The model under review builds one solid part; all positions refer to its coordinate system, in mm. Face numbers are marked on the shaded views. A direction names the side the tool comes from. Round coordinates to 2 decimals unless told otherwise and drop trailing zeros. Order: outer loops, then holes, each group sorted by start corner. A loop starts at its lowest first (then second) coordinate and runs counter-clockwise, first axis right, second up. Notation, with made-up numbers: M -34,43.25 L 0,43.25 A30 ccw 0,68.25 Z; hole C 45,-17.5 d2. An arc over 180 degrees is marked long. Use a Markdown table: item, result. Add a question column.
1. Insertion check: P1, Ø7, axis at x = -29, y = 60.5, coming from the +Z side; P2, Ø1, axis at x = -13, y = 155, coming from the -Z side; P3, Ø6.5, axis at x = 2.5, z = -15.5, coming from the +Y side; P4, Ø4, axis at y = 92, z = -23.5, coming from the -X side (1 decimal). Each pin has a flat end and moves straight along its axis. Give the tip position at first contact, or say it passes through.
2. Consider section A-A on y = 153. State the section outline as (x, z) points, then the cut area to 3 significant figures.
3. Consider section B-B on z = 17. State the section outline as (x, y) points, then the cut area to 3 significant figures.
4. For the marked faces 1, 2 and 3, list the 3-axis set-ups (+Z, -Z, +X, -X, +Y, -Y) from which the entire face can be reached by the end or side of a thin tool; tool diameter is ignored.
5. Consider section D-D on z = 0. State the section outline as (x, y) points.
6. Consider section C-C on x = 21.5. State the section outline as (y, z) points.
7. To check wall thickness, follow probe 1 along X at (y, z) = (41.5, 0); probe 2 along Y at (x, z) = (24.5, -16); probe 3 along Z at (x, y) = (0, 85). State the ranges of each line that lie inside material, in increasing order.
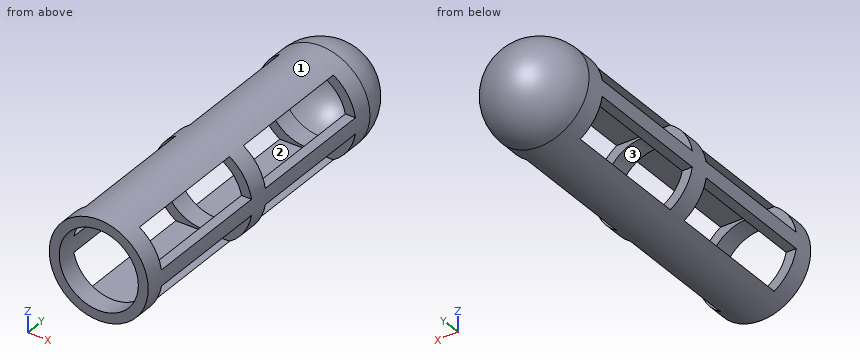
from build123d import *

# Parameters (mm, degrees)
F0_R     = 31.75
F0_R_2   = 25.4
F1_DEPTH = 203.2
F3_ANGLE = -180
F4_W     = 82.55
F4_H     = 21.59
F5_DEPTH = 63.5


with BuildPart() as f1:
    # F0 (on Front) → F1 (new body)
    with BuildSketch(Plane.XZ):
        Circle(F0_R)
        Circle(F0_R_2, mode=Mode.SUBTRACT)
    extrude(amount=-F1_DEPTH)

    # F2 (on face) → F3 (revolve)
    with BuildSketch(Plane(origin=(0, 203.2, 0), x_dir=(-1, 0, 0), z_dir=(0, 1, 0))):
        with BuildLine():
            Line((0, 25.4), (0, 31.75))
            ThreePointArc((0, 31.75), (-31.75, 0), (0, -31.75))
            Line((0, -31.75), (0, -25.4))
            ThreePointArc((0, -25.4), (-25.4, 0), (0, 25.4))
        make_face()
    revolve(axis=Axis((0, 203.2, 0), (0, 0, -1)), revolution_arc=F3_ANGLE)

    # F4 (on Right) → F5 (cut, symmetric)
    with BuildSketch(Plane.YZ):
        Polygon((190.5, 5.08), (190.5, 26.67), (133.185655, 26.67), (120.587125, 26.67), (107.95, 26.67), (107.95, 5.08), (120.587125, 5.08), (133.287125, 5.08), align=None)
        with Locations((149.225, -15.875)):
            Rectangle(F4_W, F4_H)
        with Locations((53.975, 15.875)):
            Rectangle(F4_W, F4_H)
        with Locations((53.975, -15.875)):
            Rectangle(F4_W, F4_H)
    extrude(amount=F5_DEPTH, both=True, mode=Mode.SUBTRACT)


solid = f1.part
Answer block:
| question | item | result |
|---|---|---|
| 1 | P1 | z = 5.08 |
| 1 | P2 | z = -29.19 |
| 1 | P3 | y = 232.41 |
| 1 | P4 | through |
| 2 | outline | M -31.34,-5.08 L -24.89,-5.08 A25.4 cw -24.89,5.08 L -31.34,5.08 A31.75 ccw Z; M -17.23,-26.67 A31.75 ccw 17.23,-26.67 Z; M -17.23,26.67 L 17.23,26.67 A31.75 ccw Z; M 24.89,-5.08 L 31.34,-5.08 A31.75 ccw 31.34,5.08 L 24.89,5.08 A25.4 cw Z |
| 2 | area | 367 mm^2 |
| 3 | outline | M -26.82,0 L -18.87,0 L -18.87,12.7 L -26.82,12.7 Z; M -26.82,95.25 L -18.87,95.25 L -18.87,107.95 L -26.82,107.95 Z; M -26.82,190.5 L -18.87,190.5 L -18.87,203.2 A18.87 cw 18.87,203.2 L 18.87,190.5 L 26.82,190.5 L 26.82,203.2 A26.82 ccw -26.82,203.2 Z; M 18.87,0 L 26.82,0 L 26.82,12.7 L 18.87,12.7 Z; M 18.87,95.25 L 26.82,95.25 L 26.82,107.95 L 18.87,107.95 Z |
| 3 | area | 1,180 mm^2 |
| 4 | face 1 | +Y, -Y |
| 4 | face 2 | +X, -X |
| 4 | face 3 | -Y |
| 5 | outline | M -31.75,0 L -25.4,0 L -25.4,203.2 A25.4 cw 25.4,203.2 L 25.4,0 L 31.75,0 L 31.75,203.2 A31.75 ccw -31.75,203.2 Z |
| 6 | outline | M 0,-23.36 L 12.7,-23.36 L 12.7,-13.52 L 0,-13.52 Z; M 0,13.52 L 12.7,13.52 L 12.7,23.36 L 0,23.36 Z; M 95.25,-23.36 L 107.95,-23.36 L 107.95,-13.52 L 95.25,-13.52 Z; M 95.25,13.52 L 107.95,13.52 L 107.95,23.36 L 95.25,23.36 Z; M 190.5,-23.36 L 203.2,-23.36 A23.36 ccw 203.2,23.36 L 190.5,23.36 L 190.5,13.52 L 203.2,13.52 A13.52 cw 203.2,-13.52 L 190.5,-13.52 Z |
| 7 | probe 1 | -31.75 to -25.4, 25.4 to 31.75 |
| 7 | probe 2 | 0 to 12.7, 95.25 to 107.95, 190.5 to 215.52 |
| 7 | probe 3 | -31.75 to -26.67, 26.67 to 31.75 |
